Work out the finished part from the listing and answer in its coordinate system (mm). A direction names the side the tool comes from. Round coordinates to 2 decimals unless told otherwise and drop trailing zeros. Write each loop counter-clockwise with the first axis right and the second up, starting at its lowest first coordinate (ties: lowest second). Pieces come first, ordered by that corner, then holes.
1. Straight lines are drawn through the part: probe 1 along Y at (x, z) = (-9.25, 7); probe 2 along Z at (x, y) = (0, 1.4); probe 3 along Y at (x, z) = (0.75, -7.25). For each, find the intervals that lie inside material, in ascending order.
2. Find section D-D (y = 10.25). Write down the section's boundary in (x, z).
3. Determine the mould class of faces 4 (the face through (-14.985, 27.014, -0.66)), 5 (the face through (4.127, 13.014, -4.62)), 6 (the face through (-3, 14, 0)), 7 (the face through (0, 28, 4)) for opening direction Z: pulls with the +Z half, pulls with the -Z half, needs draft (parallel to the pull), parting line crosses it, or undercut.
4. A tool of negligible diameter and unlimited length cuts with its end or side. For faces 1 (the face through (-14.985, 13.014, -0.66)), 2 (the face through (-4, 14, 4)), 3 (the face through (0.831, 0.986, -8.597)), from which of +Z, -Z, +X, -X, +Y, -Y can it reach the whole face along a straight path? Write none if from no direction.
5. Find section A-A (x = 0). Count the separate pieces of the cut face and the enclosed holes in it, and give its area (3 significant figures).
6. Find section C-C (x = -9.5). Write down the section's boundary in (y, z), and give its area (3 significant figures).
7. Flat-ended cylindrical pins translate along their axes: pin 1 Ø8 at (x, y) = (8.5, 10.5) entering from +Z; pin 2 Ø1.5 at (x, y) = (5, 22.5) entering from +Z; pin 3 Ø2.5 at (x, z) = (9.56, -9.44) entering from -Y. Find the tip coordinate at first contact, or state that the pin passes through.
Autodesk Inventor part; units mm, degrees
ref_plane "YZ Plane" through (0, 0, 0) normal (1, 0, 0) x (0, 1, 0)
ref_plane "XZ Plane" through (0, 0, 0) normal (0, 1, 0) x (-1, 0, 0)
ref_plane "XY Plane" through (0, 0, 0) normal (0, 0, 1) x (1, 0, 0)
sketch "Sketch1" plane through (0, 0, 0) normal (0, 0, 1) x (1, 0, 0)
  line L0 (0, 24) -> (0, 0)
  line L1 (3, 0) -> (3, 28)
  line L2 (3, 0) -> (12, 0)
  line L3 (12, 0) -> (12, 2)
  line L4 (12, 2) -> (5, 2)
  line L5 (5, 2) -> (5, 12)
  line L6 (5, 12) -> (15, 12)
  line L7 (15, 12) -> (15, 14)
  line L8 (15, 14) -> (5, 14)
  line L9 (5, 14) -> (5, 26)
  line L10 (5, 26) -> (15, 26)
  line L11 (15, 26) -> (15, 28)
  line L12 (15, 28) -> (3, 28)
  dimension "d1" = 6
  dimension "d2" = 9
  dimension "d3" = 2
  dimension "d4" = 7
  dimension "d5" = 2
  dimension "d6" = 10
  dimension "d7" = 2
  dimension "d8" = 2
  dimension "d9" = 28
  dimension "d10" = 12
  dimension "d11" = 10
  dimension "d17" = 26
  dimension "d18" = 2
revolve "Revolution1" add sketch "Sketch1" angle 360 about axis through (0, 24, 0) along (0, -1, 0)
sketch "Sketch2" plane through (0, 0, 0) normal (0, -1, 0) x (1, 0, 0)
  circle A0 centre (0, -7) radius 1.8
  circle A1 centre (7, 0) radius 1.8
  circle A2 centre (0, 7) radius 1.8
  circle A3 centre (-7, 0) radius 1.8
  point P0 (0, 0)
  dimension "d20" = 3.6
  dimension "d21" = 7
  dimension "d24" = 360
extrude "Extrusion1" cut sketch "Sketch2" against normal blind 2
sketch "Sketch3" plane through (0, 12, 0) normal (0, -1, 0) x (1, 0, 0)
  point P0 (0, 0)
  point P1 (3.3947, -4.7826)
hole "Hole1" at (3.3947, 12, -4.7826) direction (0, 1, 0) diameter 1.5 depth 2
sketch "Sketch4" plane through (0, 12, 0) normal (0, -1, 0) x (1, 0, 0)
  point P0 (0, 0)
  point P1 (9.5617, -9.4421)
hole "Hole2" at (9.5617, 12, -9.4421) direction (0, 1, 0) diameter 1.5 depth 2
properties part number "SpoolMk2"
Worked answers:
1. probe 1: y = 0 to 2, 12 to 14, 26 to 28
1. probe 2: z = -12 to -8.8, -5.2 to -3, 3 to 5.2, 8.8 to 12
1. probe 3: y = 12 to 14, 26 to 28
2. outline: circle Ø10 at (0, 0); hole circle Ø6 at (0, 0)
3. face 4: parting line crosses it
3. face 5: undercut
3. face 6: undercut
3. face 7: needs draft
4. face 1: +Y, -Y
4. face 2: none
4. face 3: -Y
5. separate pieces: 4
5. enclosed holes: 0
5. area: 206 mm2
6. outline: (0, -7.33) - (2, -7.33) - (2, 7.33) - (0, 7.33) - close; (12, -11.61) - (14, -11.61) - (14, 11.61) - (12, 11.61) - close; (26, -11.61) - (28, -11.61) - (28, 11.61) - (26, 11.61) - close
6. area: 122 mm2
7. pin 1: stops at z = 14.21
7. pin 2: stops at z = 2.63
7. pin 3: stops at y = 12
